Autodesk Inventor part; units mm, degrees
ref_plane "РабПлоскость1" through (-81.2124, 0, 0) normal (0, -1, 0) x (1, 0, 0)
ref_plane "YZ Plane" through (0, 0, 0) normal (1, 0, 0) x (0, 1, 0)
ref_plane "XZ Plane" through (0, 0, 0) normal (0, 1, 0) x (-1, 0, 0)
sketch "Эскиз1" plane through (0, 0, 0) normal (0, 0, 1) x (1, 0, 0)
  line L0 (-100, -75) -> (100, -75)
  line L1 (100, -75) -> (100, 75)
  line L2 (100, 75) -> (-100, 75)
  line L3 (-100, 75) -> (-100, -75)
  line L4 (-100, -75) -> (100, 75) construction
  line L5 (100, -75) -> (-100, 75) construction
  point P0 (0, 0)
  dimension "d0" = 200
  dimension "d1" = 150
extrude "Выдавливание1" add sketch "Эскиз1" along normal blind 5
sketch "Эскиз2" plane through (0, 0, 5) normal (0, 0, 1) x (1, 0, 0)
  line L0 (-100, -75) -> (100, -75)
  line L1 (100, -75) -> (100, 75)
  line L2 (100, 75) -> (-100, 75)
  line L3 (-100, 75) -> (-100, -75)
  line L4 (100, 75) -> (-100, 75) construction
  line L5 (0, 75) -> (0, -75) construction
  line L6 (-100, 0) -> (100, 0) construction
  line L7 (100, -75) -> (100, 75) construction
  line L8 (-100, -12.5) -> (100, -12.5) construction
  line L9 (100, -12.5) -> (100, 12.5) construction
  line L10 (100, 12.5) -> (-100, 12.5) construction
  line L11 (-100, 12.5) -> (-100, -12.5) construction
  line L12 (-100, -12.5) -> (100, 12.5) construction
  line L13 (100, -12.5) -> (-100, 12.5) construction
  line L14 (-100, 0) -> (0, 0) construction
  line L15 (-51.2124, 75) -> (-51.2124, -75) construction
  line L16 (-100, -75) -> (100, -75) construction
  line L17 (0, 0) -> (100, 0) construction
  line L18 (50, 75) -> (50, -75) construction
  line L19 (-81.2124, -12.5) -> (-21.2124, -12.5)
  line L20 (-21.2124, -12.5) -> (-21.2124, 12.5)
  line L21 (-21.2124, 12.5) -> (-81.2124, 12.5)
  line L22 (-81.2124, 12.5) -> (-81.2124, -12.5)
  line L23 (-81.2124, -12.5) -> (-21.2124, 12.5) construction
  line L24 (-21.2124, -12.5) -> (-81.2124, 12.5) construction
  line L25 (81.2124, -12.5) -> (21.2124, -12.5)
  line L26 (21.2124, -12.5) -> (21.2124, 12.5)
  line L27 (21.2124, 12.5) -> (81.2124, 12.5)
  line L28 (81.2124, 12.5) -> (81.2124, -12.5)
  point P0 (-51.2124, 0)
  dimension "d4" = 25
  dimension "d5" = 60
extrude "Выдавливание2" cut sketch "Эскиз2" against normal blind 5 contours L22 L21 L20 L19 | L25 L26 L27 L28
sketch "Эскиз3" plane through (-81.2124, 12.5, 5) normal (0, -1, 0) x (1, 0, 0)
  line L0 (0, 0) -> (60, 0)
  line L1 (30, 0) -> (30, 14.9537) construction
  line L2 (30, 0) -> (40, 0) construction
  line L3 (30, 0) -> (35, 0) construction
  line L4 (30, 0) -> (25, 0) construction
  line L5 (25, 0) -> (35, 0) construction
  line L6 (25, 0) -> (35, 0)
  line L7 (30, 0) -> (30, 3) construction
  circle A0 centre (30, 1.5) radius 1.5
  arc A1 (32.3946, 0.7816) -> (27.6054, 0.7816) centre (30, 1.5) ccw
  line L8 (35, 0) -> (32.3946, 0.7816)
  line L9 (25, 0) -> (27.6054, 0.7816)
  point P0 (81.2124, -5)
  dimension "d8" = 10
  dimension "d9" = 5
  dimension "d10" = 5
  dimension "d11" = 3
  dimension "d12" = 1
extrude "Выдавливание3" add sketch "Эскиз3" against normal blind 5
mirror "Зеркальное отражение1" about plane through (0, 0, 0) normal (0, 1, 0) of "Выдавливание3"
sketch "Эскиз4" plane through (-81.2124, 12.5, 0) normal (0, -1, 0) x (1, 0, 0)
  circle A0 centre (30, 6.5) radius 1.5
  point P0 (81.2124, 0)
surface extrude "ВыдавПврх1" sketch "Эскиз4" along normal up to next shown yes curves A0
boundary_patch "Участок поверхности1"
boundary_patch "Участок поверхности2"
ref_plane "РабПлоскость1" through (-81.2124, 0, 0) normal (0, -1, 0) x (1, 0, 0)
sketch "Эскиз6" plane through (0, 0, 5) normal (0, 0, 1) x (1, 0, 0)
  line L0 (81.2124, -12.5) -> (21.2124, -12.5)
  line L1 (21.2124, -12.5) -> (21.2124, 12.5)
  line L2 (21.2124, 12.5) -> (81.2124, 12.5)
  line L3 (81.2124, 12.5) -> (81.2124, -12.5)
  line L4 (-100, -75) -> (100, -75)
  line L5 (100, -75) -> (100, 75)
  line L6 (100, 75) -> (-100, 75)
  line L7 (-100, 75) -> (-100, -75)
  line L8 (-46.2124, -12.5) -> (-46.2124, -17.5)
  line L9 (-46.2124, -17.5) -> (-51.2124, -17.5)
  line L10 (-51.2124, -17.5) -> (-56.2124, -17.5)
  line L11 (-56.2124, -17.5) -> (-56.2124, -12.5)
  line L12 (-56.2124, -12.5) -> (-81.2124, -12.5)
  line L13 (-81.2124, -12.5) -> (-81.2124, 12.5)
  line L14 (-81.2124, 12.5) -> (-56.2124, 12.5)
  line L15 (-56.2124, 12.5) -> (-56.2124, 17.5)
  line L16 (-56.2124, 17.5) -> (-51.2124, 17.5)
  line L17 (-51.2124, 17.5) -> (-46.2124, 17.5)
  line L18 (-46.2124, 17.5) -> (-46.2124, 12.5)
  line L19 (-46.2124, 12.5) -> (-21.2124, 12.5)
  line L20 (-21.2124, 12.5) -> (-21.2124, -12.5)
  line L21 (-21.2124, -12.5) -> (-46.2124, -12.5)
  line L22 (-100, -75) -> (100, -75) construction
  line L23 (-21.2124, -75) -> (-21.2124, 75) construction
  line L24 (100, 75) -> (-100, 75) construction
  line L25 (-21.2124, 12.5) -> (-21.2124, 75) construction
  line L26 (-21.2124, 75) -> (21.2124, 75) construction
  line L27 (21.2124, 75) -> (21.2124, 12.5) construction
  line L28 (21.2124, 12.5) -> (-21.2124, 12.5) construction
  line L29 (-21.2124, 12.5) -> (-21.2124, 75) construction
  line L30 (-21.2124, -75) -> (21.2124, -75) construction
  line L31 (21.2124, -75) -> (21.2124, -12.5) construction
  line L32 (21.2124, -12.5) -> (-21.2124, -12.5) construction
  line L33 (-21.2124, -12.5) -> (-21.2124, -75) construction
  line L34 (100, -75) -> (100, 75) construction
  line L35 (-100, -7.5) -> (100, -7.5) construction
  line L36 (100, -7.5) -> (100, 7.5) construction
  line L37 (100, 7.5) -> (-100, 7.5) construction
  line L38 (-100, 7.5) -> (-100, -7.5) construction
  line L39 (-100, -7.5) -> (100, 7.5) construction
  line L40 (100, -7.5) -> (-100, 7.5) construction
  line L41 (0, 7.5) -> (0, 17.5) construction
  line L42 (0, -7.5) -> (0, -28.0993) construction
  line L43 (-21.2124, 0) -> (21.2124, 0) construction
  arc A0 (-5, -38.0993) -> (5, -38.0993) centre (0, -38.0993) ccw
  arc A1 (5, -7.5) -> (-5, -7.5) centre (0, -7.5) ccw
  line L44 (-5, -7.5) -> (-5, -38.0993)
  line L45 (5, -38.0993) -> (5, -7.5)
  line L46 (100, 0) -> (-100, 0) construction
  line L47 (-100, 75) -> (-100, -75) construction
  arc A2 (5, 38.0993) -> (-5, 38.0993) centre (0, 38.0993) ccw
  arc A3 (-5, 7.5) -> (5, 7.5) centre (0, 7.5) ccw
  line L48 (-5, 7.5) -> (-5, 38.0993)
  line L49 (5, 38.0993) -> (5, 7.5)
  point P0 (0, 0)
  point P1 (0, -17.7997)
  dimension "d24" = 15
  dimension "d25" = 10
  dimension "d38" = 10
  dimension "d39" = 10
extrude "Выдавливание5" cut sketch "Эскиз6" against normal blind 20 contours L44 A1 L45 A0 | L49 A3 L48 A2
mirror "Зеркальное отражение2" about plane through (0, 0, 0) normal (1, 0, 0) of "Выдавливание3", "ВыдавПврх1", "Зеркальное отражение1"
sketch "Эскиз7" plane through (0, 0, 5) normal (0, 0, 1) x (1, 0, 0)
  line L0 (-100, -75) -> (100, -75)
  line L1 (100, -75) -> (100, 75)
  line L2 (100, 75) -> (-100, 75)
  line L3 (-100, 75) -> (-100, -75)
  line L4 (-46.2124, -12.5) -> (-46.2124, -17.5)
  line L5 (-46.2124, -17.5) -> (-51.2124, -17.5)
  line L6 (-51.2124, -17.5) -> (-56.2124, -17.5)
  line L7 (-56.2124, -17.5) -> (-56.2124, -12.5)
  line L8 (-56.2124, -12.5) -> (-81.2124, -12.5)
  line L9 (-81.2124, -12.5) -> (-81.2124, 12.5)
  line L10 (-81.2124, 12.5) -> (-56.2124, 12.5)
  line L11 (-56.2124, 12.5) -> (-56.2124, 17.5)
  line L12 (-56.2124, 17.5) -> (-51.2124, 17.5)
  line L13 (-51.2124, 17.5) -> (-46.2124, 17.5)
  line L14 (-46.2124, 17.5) -> (-46.2124, 12.5)
  line L15 (-46.2124, 12.5) -> (-21.2124, 12.5)
  line L16 (-21.2124, 12.5) -> (-21.2124, -12.5)
  line L17 (-21.2124, -12.5) -> (-46.2124, -12.5)
  line L18 (56.2124, -12.5) -> (56.2124, -17.5)
  line L19 (56.2124, -17.5) -> (51.2124, -17.5)
  line L20 (51.2124, -17.5) -> (46.2124, -17.5)
  line L21 (46.2124, -17.5) -> (46.2124, -12.5)
  line L22 (46.2124, -12.5) -> (21.2124, -12.5)
  line L23 (21.2124, -12.5) -> (21.2124, 12.5)
  line L24 (21.2124, 12.5) -> (46.2124, 12.5)
  line L25 (46.2124, 12.5) -> (46.2124, 17.5)
  line L26 (46.2124, 17.5) -> (51.2124, 17.5)
  line L27 (51.2124, 17.5) -> (56.2124, 17.5)
  line L28 (56.2124, 17.5) -> (56.2124, 12.5)
  line L29 (56.2124, 12.5) -> (81.2124, 12.5)
  line L30 (81.2124, 12.5) -> (81.2124, -12.5)
  line L31 (81.2124, -12.5) -> (56.2124, -12.5)
  line L32 (-100, 75) -> (-70, 75) construction
  line L33 (-70, 75) -> (-70, 45) construction
  line L34 (-70, 45) -> (-100, 45) construction
  line L35 (-100, 45) -> (-100, 75) construction
  circle A0 centre (-70, 45) radius 5
  line L36 (100, -75) -> (100, 75) construction
  line L37 (100, 0) -> (-100, 0) construction
  line L38 (100, 75) -> (-100, 75) construction
  line L39 (0, 75) -> (0, -75) construction
  line L40 (-100, -75) -> (100, -75) construction
  circle A1 centre (70, 45) radius 5
  line L41 (-100, -75) -> (100, -75)
  line L42 (-70, -75) -> (-70, -35) construction
  line L43 (-70, -35) -> (-100, -35) construction
  circle A2 centre (-70, -35) radius 5
  line L44 (70, -75) -> (70, -35) construction
  line L45 (70, -35) -> (100, -35) construction
  circle A3 centre (70, -35) radius 5
  line L46 (-100, -75) -> (-100, -55)
  line L47 (-100, -55) -> (100, -55)
  line L48 (100, -75) -> (100, -55)
  point P0 (0, 0)
  dimension "d30" = 30
  dimension "d31" = 30
  dimension "d32" = 10
  dimension "d35" = 40
  dimension "d36" = 10
  dimension "d37" = 20
extrude "Выдавливание6" cut sketch "Эскиз7" against normal blind 20 contours L3 L47 L1 L0 | A0 | A1 | A2 | A3
properties part number "Down"
Model file for the job. Use its own axes, mm. A direction names the side the tool comes from. Coordinates: 2 decimals unless noted, no trailing zeros. Order: outer loops, then holes, each group sorted by start corner. A loop starts at its lowest first (then second) coordinate and runs counter-clockwise, first axis right, second up. Notation, with made-up numbers: (-11.5, 10.25) -> (27.5, 10.25) arc R16 cw to (27.5, 36.25) -> close; hole circle Ø11 at (50, 8.5). An arc over 180 degrees is marked (long way). Answer as a JSON object with one key per item and string values. Group by question number.
1) Cut at C-C, the plane z = 3.5. Count the separate pieces of the cut face and the enclosed holes in it, then the cut area to 3 significant figures.
2) Pull direction Y, two halves, no side cores. Call faces 4 (the face through (21, 11, 5)), 5 (the face through (-21.212, 0, 3)), 6 (the face through (-52, 17.5, 8)): +Y half, -Y half, draft (parallel to the pull), parting line (faces both ways), or undercut.
3) Cut at B-B, the plane y = 26. Write the cut outline in (x, z), then the cut area to 3 significant figures.
4) Cut at D-D, the plane y = -35. Write the cut outline in (x, z).
5) Which spindle directions (+Z, -Z, +X, -X, +Y, -Y) get a long thin tool onto all of the face, cutting with end or side? Do faces 1 (the face through (50, 17.5, 8)), 2 (the face through (-81.212, 0, 3)), 3 (the face through (-51.15, 14.96, 9)). Say none if no direction does.
6) Cut at A-A, the plane x = -42. Write the cut outline in (y, z).
7) Flat gauge pins, fed straight in: pin 1 (1.8 mm diameter, centred on x = -51.21, z = 6.5, fed in from -Y) (3 decimals); pin 2 (1.5 mm diameter, centred on x = -36, y = 16, fed in from +Z). Where does each tip first touch, or does it go through?
8) Drill centre lines: L1, parallel to X at y = -10.5, z = 0.75; L2, parallel to X at y = 15, z = 6.5; L3, parallel to Y at x = 70, z = 1.9. Where is each one in solid material? Low to high.
Check values:
{
 "1": {"separate pieces": "1", "enclosed holes": "8", "area": "21,900 mm²"},
 "2": {"face 4": "draft", "face 5": "undercut", "face 6": "+Y half"},
 "3": {"outline": "(-100, 0) -> (-5, 0) -> (-5, 5) -> (-100, 5) -> close; (5, 0) -> (100, 0) -> (100, 5) -> (5, 5) -> close", "area": "950 mm²"},
 "4": {"outline": "(-100, 0) -> (-75, 0) -> (-75, 5) -> (-100, 5) -> close; (-65, 0) -> (-5, 0) -> (-5, 5) -> (-65, 5) -> close; (5, 0) -> (65, 0) -> (65, 5) -> (5, 5) -> close; (75, 0) -> (100, 0) -> (100, 5) -> (75, 5) -> close"},
 "5": {"face 1": "+Z, +X, -X, +Y", "face 2": "+Z, -Z", "face 3": "+Y, -Y"},
 "6": {"outline": "(-55, 0) -> (-12.5, 0) -> (-12.5, 5) -> (-55, 5) -> close; (12.5, 0) -> (75, 0) -> (75, 5) -> (12.5, 5) -> close"},
 "7": {"pin 1": "passes through", "pin 2": "stops at z = 5"},
 "8": {"L1": "x = -100 to -81.21, -21.21 to -5, 5 to 21.21, 81.21 to 100", "L2": "x = -53.71 to -52.71, -49.71 to -48.71, 48.71 to 49.71, 52.71 to 53.71", "L3": "y = -55 to -40, -30 to -12.5, 12.5 to 40, 50 to 75"}
}
